```python
from build123d import *

# Parameters (mm, degrees)
F0_W     = 81.28
F0_H     = 144.272
F1_DEPTH = 4.7752
F2_W     = 43.18
F2_H     = 118.872
F3_DEPTH = 25.4
F4_SIZE  = 10.16


with BuildPart() as f1:
    # F0 (on Top) → F1 (new body)
    with BuildSketch(Plane.XY):
        with Locations((-2.556553, 4.684015)):
            Rectangle(F0_W, F0_H)
    extrude(amount=F1_DEPTH)

    # F2 (on face) → F3 (cut)
    with BuildSketch(Plane.XY.offset(4.7752)):
        with Locations((-2.556553, 4.684015)):
            Rectangle(F2_W, F2_H)
    extrude(amount=-F3_DEPTH, mode=Mode.SUBTRACT)

    # F4
    f4_edges = [f1.edges().sort_by_distance(p)[0] for p in [
        (38.083447, -67.451985, 2.3876),
        (-43.196553, -67.451985, 2.3876),
        (38.083447, 76.820015, 2.3876),
        (-43.196553, 76.820015, 2.3876),
    ]]
    chamfer(f4_edges, length=F4_SIZE)


solid = f1.part
```
The model under review builds one solid part; all positions refer to its coordinate system, in mm. A direction names the side the tool comes from. Round coordinates to 2 decimals unless told otherwise and drop trailing zeros. Loops run counter-clockwise (first coordinate to the right, second up) from the corner with the lowest first, then second, coordinate; pieces in that order, holes last. Notation, with made-up numbers: (14, 29.25) -> (67, 29.25) arc R6 cw to (67, 37.25) -> close; hole circle Ø5 at (58.25, -15.5). An arc over 180 degrees is marked (long way). Answer as a JSON object with one key per item and string values. Group by question number.
1) We need section A-A on y = 3.5. Write out the cut boundary in (x, z).
2) Mouldability with a two-part tool opening along X and no side actions: class faces 3 (the face through (-3, -54.752, 2)), 4 (the face through (-38.05, -62.44, 2.35)), 5 (the face through (33.075, -62.301, 2.354)), 6 (the face through (-30, 6, 4.775)) as released by +X, released by -X, zero draft, split by the parting line, or undercut.
3) For faces 1 (the face through (-3, 64.12, 2)), 2 (the face through (-3, 76.82, 2)), list the 3-axis set-ups (+Z, -Z, +X, -X, +Y, -Y) from which the entire face can be reached by the end or side of a thin tool; tool diameter is ignored.
4) We need section D-D on x = 32. Write out the cut boundary in (y, z), then the cut area to 3 significant figures.
5) We need section B-B on z = 3.5. Write out the cut boundary in (x, y), then the cut area to 3 significant figures.
6) We need section C-C on x = -36.5. Write out the cut boundary in (y, z).
7) For line 1 (X direction, y = 62.5, z = 0.8); line 2 (Y direction, x = -9.5, z = 0.3); line 3 (Y direction, x = -34.5, z = 4.3), list the stretches that pass through material, from the lowest coordinate up. Write a range as [from, to].
Result set:
{
 "1": {"outline": "(-43.2, 0) -> (-24.15, 0) -> (-24.15, 4.78) -> (-43.2, 4.78) -> close; (19.03, 0) -> (38.08, 0) -> (38.08, 4.78) -> (19.03, 4.78) -> close"},
 "2": {"face 3": "undercut", "face 4": "released by -X", "face 5": "released by +X", "face 6": "zero draft"},
 "3": {"face 1": "+Z, -Z", "face 2": "+Z, -Z, +X, -X, +Y"},
 "4": {"outline": "(-63.38, 0) -> (72.74, 0) -> (72.74, 4.78) -> (-63.38, 4.78) -> close", "area": "650 mm²"},
 "5": {"outline": "(-43.2, -57.29) -> (-33.04, -67.45) -> (27.92, -67.45) -> (38.08, -57.29) -> (38.08, 66.66) -> (27.92, 76.82) -> (-33.04, 76.82) -> (-43.2, 66.66) -> close; hole (-24.15, -54.75) -> (19.03, -54.75) -> (19.03, 64.12) -> (-24.15, 64.12) -> close", "area": "6,390 mm²"},
 "6": {"outline": "(-63.99, 0) -> (73.36, 0) -> (73.36, 4.78) -> (-63.99, 4.78) -> close"},
 "7": {"line 1": "[-43.2, -24.15], [19.03, 38.08]", "line 2": "[-67.45, -54.75], [64.12, 76.82]", "line 3": "[-65.99, 75.36]"}
}
